Check sheet for the modelled part. Datum: model origin and axes. Units: mm. Face numbers are marked on the shaded views. Give positions to 0.01 mm unless a question says otherwise; leave off trailing zeros. Loops run counter-clockwise (first coordinate to the right, second up) from the corner with the lowest first, then second, coordinate; pieces in that order, holes last. Notation, with made-up numbers: M 56,53.5 L 61,53.5 A22 cw 61,74.5 Z; hole C 36,76.25 d10. An arc over 180 degrees is marked long. Write each question's results on one line, items separated by ' | '. Start each with the question number.
1. Sectioned sample at B-B on y = 5. Record the cut outline in (x, z), and give its area (3 significant figures).
2. Draft check along Z on the marked faces 1, 2 and 3. Enter one of: pulls with the +Z half, pulls with the -Z half, needs draft (parallel to the pull), parting line crosses it, or undercut.
3. Material ranges on line 1 along X through (y, z) = (5.75, 0); line 2 along Z through (x, y) = (0, 0.3); line 3 along X through (y, z) = (0.75, 0), recorded low to high.
4. Sectioned sample at C-C on x = 13.5. Record the cut outline in (y, z), and give its area (3 significant figures).
5. Sectioned sample at A-A on z = 10. Record the cut outline in (x, y).
6. Go/stop test with flat-tipped pins: pin 1 (1.5 mm diameter, centred on x = 59.5, z = 34.5, fed in from -Y); pin 2 (0.8 mm diameter, centred on y = 15, z = 63, fed in from +X); pin 3 (1.3 mm diameter, centred on y = 13, z = 63, fed in from -X). Record where each tip stops, or that it passes through.
```python
from build123d import *

# Parameters (mm, degrees)
SKETCH_1_R          = 71.5
SKETCH_1_R_2        = 70
EXTRUDE_1_DEPTH     = 19
SKETCH_2_R          = 71.5
SKETCH_2_R_2        = 65.25
EXTRUDE_2_DEPTH     = 1
CUT_EXTRUDE_1_DEPTH = 10
EXTRUDE_4_DEPTH     = 2
CUT_EXTRUDE_2_DEPTH = 0.2


with BuildPart() as part:
    # 草图1 → 凸台-拉伸1 (new body)
    with BuildSketch(Plane(origin=(0, 0, 0), x_dir=(1, 0, 0), z_dir=(0, 1, 0))):
        Circle(SKETCH_1_R)
        Circle(SKETCH_1_R_2, mode=Mode.SUBTRACT)
    extrude(amount=EXTRUDE_1_DEPTH)

    # 草图2 → 凸台-拉伸2 (add)
    with BuildSketch(Plane.XZ):
        Circle(SKETCH_2_R)
        Circle(SKETCH_2_R_2, mode=Mode.SUBTRACT)
    extrude(amount=-EXTRUDE_2_DEPTH)

    # 草图4 → 切除-拉伸1 (cut)
    with BuildSketch(Plane(origin=(0, 19, 0), x_dir=(1, 0, 0), z_dir=(0, 1, 0))):
        Polygon((-31.5, 0), (-31.5, -83.475080556), (0, -83.475080556), (31.5, -83.475080556), (31.5, 0), align=None)
    extrude(amount=-CUT_EXTRUDE_1_DEPTH, mode=Mode.SUBTRACT)

    # 草图5 → 凸台-拉伸4 (add)
    with BuildSketch(Plane.XZ):
        with BuildLine():
            Line((6, 71.247806984), (6, 91.247806984))
            Line((6, 91.247806984), (-6, 91.247806984))
            Line((-6, 91.247806984), (-6, 71.247806984))
            ThreePointArc((-6, 71.247806984), (0, 71.5), (6, 71.247806984))
        make_face()
    extrude(amount=-EXTRUDE_4_DEPTH)

    # 草图6 → 切除-拉伸2 (cut)
    with BuildSketch(Plane.XZ):
        with BuildLine():
            Line((-1, -65.242336715), (-1, -71.493006651))
            ThreePointArc((-1, -71.493006651), (0, -71.5), (1, -71.493006651))
            Line((1, -71.493006651), (1, -65.242336715))
            ThreePointArc((1, -65.242336715), (0, -65.25), (-1, -65.242336715))
        make_face()
        with BuildLine():
            Line((1, -65.242336715), (-1, -65.242336715))
            ThreePointArc((-1, -65.242336715), (0, -65.25), (1, -65.242336715))
        make_face()
        with BuildLine():
            Line((-33.487193761, -56.001520997), (-36.612528729, -61.414759953))
            ThreePointArc((-36.612528729, -61.414759953), (-35.75, -61.920816371), (-34.880477922, -62.414759953))
            Line((-34.880477922, -62.414759953), (-31.755142954, -57.001520997))
            ThreePointArc((-31.755142954, -57.001520997), (-32.625, -56.508157597), (-33.487193761, -56.001520997))
        make_face()
        with BuildLine():
            Line((-57.001520997, -31.755142954), (-62.414759953, -34.880477922))
            ThreePointArc((-62.414759953, -34.880477922), (-61.920816371, -35.75), (-61.414759953, -36.612528729))
            Line((-61.414759953, -36.612528729), (-56.001520997, -33.487193761))
            ThreePointArc((-56.001520997, -33.487193761), (-56.508157597, -32.625), (-57.001520997, -31.755142954))
        make_face()
        with BuildLine():
            Line((-65.242336715, 1), (-71.493006651, 1))
            ThreePointArc((-71.493006651, 1), (-71.5, 0), (-71.493006651, -1))
            Line((-71.493006651, -1), (-65.242336715, -1))
            ThreePointArc((-65.242336715, -1), (-65.25, 0), (-65.242336715, 1))
        make_face()
        with BuildLine():
            Line((-56.001520997, 33.487193761), (-61.414759953, 36.612528729))
            ThreePointArc((-61.414759953, 36.612528729), (-61.920816371, 35.75), (-62.414759953, 34.880477922))
            Line((-62.414759953, 34.880477922), (-57.001520997, 31.755142954))
            ThreePointArc((-57.001520997, 31.755142954), (-56.508157597, 32.625), (-56.001520997, 33.487193761))
        make_face()
        with BuildLine():
            Line((-31.755142954, 57.001520997), (-34.880477922, 62.414759953))
            ThreePointArc((-34.880477922, 62.414759953), (-35.75, 61.920816371), (-36.612528729, 61.414759953))
            Line((-36.612528729, 61.414759953), (-33.487193761, 56.001520997))
            ThreePointArc((-33.487193761, 56.001520997), (-32.625, 56.508157597), (-31.755142954, 57.001520997))
        make_face()
        with BuildLine():
            Line((1, 65.242336715), (1, 71.493006651))
            ThreePointArc((1, 71.493006651), (0, 71.5), (-1, 71.493006651))
            Line((-1, 71.493006651), (-1, 65.242336715))
            ThreePointArc((-1, 65.242336715), (0, 65.25), (1, 65.242336715))
        make_face()
        with BuildLine():
            Line((33.487193761, 56.001520997), (36.612528729, 61.414759953))
            ThreePointArc((36.612528729, 61.414759953), (35.75, 61.920816371), (34.880477922, 62.414759953))
            Line((34.880477922, 62.414759953), (31.755142954, 57.001520997))
            ThreePointArc((31.755142954, 57.001520997), (32.625, 56.508157597), (33.487193761, 56.001520997))
        make_face()
        with BuildLine():
            Line((57.001520997, 31.755142954), (62.414759953, 34.880477922))
            ThreePointArc((62.414759953, 34.880477922), (61.920816371, 35.75), (61.414759953, 36.612528729))
            Line((61.414759953, 36.612528729), (56.001520997, 33.487193761))
            ThreePointArc((56.001520997, 33.487193761), (56.508157597, 32.625), (57.001520997, 31.755142954))
        make_face()
        with BuildLine():
            Line((65.242336715, -1), (71.493006651, -1))
            ThreePointArc((71.493006651, -1), (71.5, 0), (71.493006651, 1))
            Line((71.493006651, 1), (65.242336715, 1))
            ThreePointArc((65.242336715, 1), (65.25, 0), (65.242336715, -1))
        make_face()
        with BuildLine():
            Line((56.001520997, -33.487193761), (61.414759953, -36.612528729))
            ThreePointArc((61.414759953, -36.612528729), (61.920816371, -35.75), (62.414759953, -34.880477922))
            Line((62.414759953, -34.880477922), (57.001520997, -31.755142954))
            ThreePointArc((57.001520997, -31.755142954), (56.508157597, -32.625), (56.001520997, -33.487193761))
        make_face()
        with BuildLine():
            Line((31.755142954, -57.001520997), (34.880477922, -62.414759953))
            ThreePointArc((34.880477922, -62.414759953), (35.75, -61.920816371), (36.612528729, -61.414759953))
            Line((36.612528729, -61.414759953), (33.487193761, -56.001520997))
            ThreePointArc((33.487193761, -56.001520997), (32.625, -56.508157597), (31.755142954, -57.001520997))
        make_face()
    extrude(amount=-CUT_EXTRUDE_2_DEPTH, mode=Mode.SUBTRACT)


solid = part.part
```
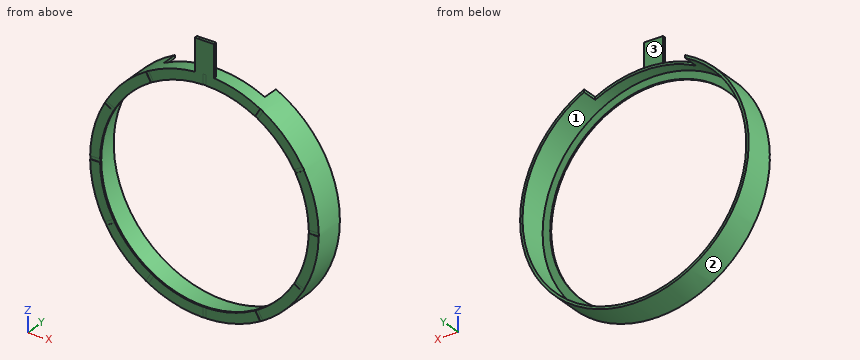
Output values:
1) outline: C 0,0 d143; hole C 0,0 d140 | area: 667 mm2
2) face 1: undercut | face 2: parting line crosses it | face 3: needs draft
3) line 1: -71.5 to -70, 70 to 71.5 | line 2: -71.5 to -65.25, 65.25 to 91.25 | line 3: -71.5 to -65.25, 65.25 to 71.5
4) outline: M 0,-70.21 L 19,-70.21 L 19,-68.69 L 1,-68.69 L 1,-63.84 L 0,-63.84 Z; M 0,63.84 L 1,63.84 L 1,68.69 L 9,68.69 L 9,70.21 L 0,70.21 Z | area: 52.5 mm2
5) outline: M -70.8,0 L -64.48,0 L -64.48,1 L -69.28,1 L -69.28,19 L -70.8,19 Z; M 64.48,0 L 70.8,0 L 70.8,19 L 69.28,19 L 69.28,1 L 64.48,1 Z
6) pin 1: y = 0.2 | pin 2: x = 34.55 | pin 3: x = -35
